The figure shows three views and two pictorial views of one solid part (mm, origin at its lowest corner). Answer the questions. A direction names the side the tool comes from. Coordinates: 2 decimals unless noted, no trailing zeros. Order: outer loops, then holes, each group sorted by start corner. A loop starts at its lowest first (then second) coordinate and runs counter-clockwise, first axis right, second up. Notation, with made-up numbers: (-35.75, 58.5) -> (10.25, 58.5) arc R29 cw to (10.25, 89.5) -> close; hole circle Ø8 at (-15.75, 75.5). An arc over 180 degrees is marked (long way). Return JSON: item names as keys, results as strings.
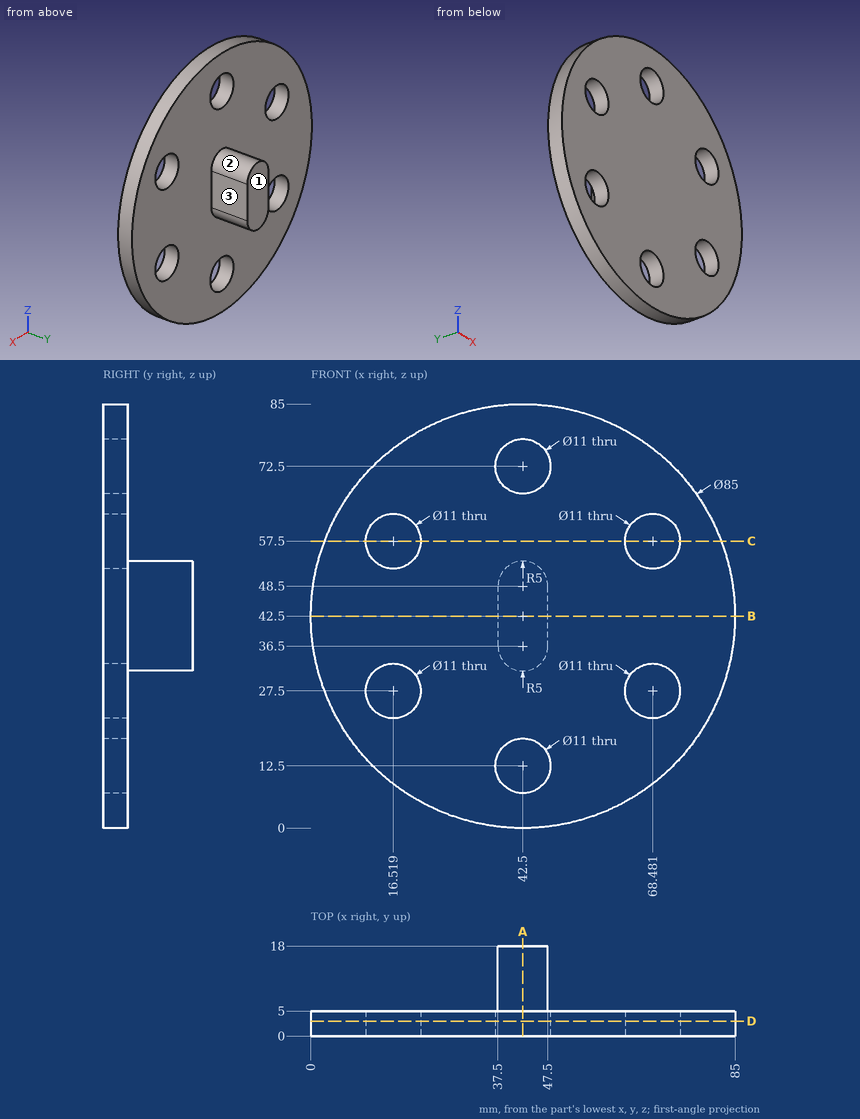
Item 1: The part is cut by section A-A on x = 42.5. Determine the outline of the cut face in (y, z), plus the area to 3 significant figures.
Answer list:
{"outline": "(0, 0) -> (5, 0) -> (5, 7) -> (0, 7) -> close; (0, 18) -> (5, 18) -> (5, 31.5) -> (18, 31.5) -> (18, 53.5) -> (5, 53.5) -> (5, 67) -> (0, 67) -> close; (0, 78) -> (5, 78) -> (5, 85) -> (0, 85) -> close", "area": "601 mm2"}
Item 2: The part is cut by section B-B on z = 42.5. Determine the outline of the cut face in (x, y), plus the area to 3 significant figures.
Answer list:
{"outline": "(0, 0) -> (85, 0) -> (85, 5) -> (47.5, 5) -> (47.5, 18) -> (37.5, 18) -> (37.5, 5) -> (0, 5) -> close", "area": "555 mm2"}
Item 3: The part is cut by section D-D on y = 3. Determine the outline of the cut face in (x, z), plus the area to 3 significant figures.
Answer list:
{"outline": "circle Ø85 at (42.5, 42.5); hole circle Ø11 at (16.52, 27.5); hole circle Ø11 at (16.52, 57.5); hole circle Ø11 at (42.5, 12.5); hole circle Ø11 at (42.5, 72.5); hole circle Ø11 at (68.48, 27.5); hole circle Ø11 at (68.48, 57.5)", "area": "5,100 mm2"}
Item 4: The part is cut by section C-C on z = 57.5. Determine the outline of the cut face in (x, y) (1 decimal).
Answer list:
{"outline": "(2.7, 0) -> (11, 0) -> (11, 5) -> (2.7, 5) -> close; (22, 0) -> (63, 0) -> (63, 5) -> (22, 5) -> close; (74, 0) -> (82.3, 0) -> (82.3, 5) -> (74, 5) -> close"}
Item 5: Flat-ended cylindrical pins translate along their axes: pin 1 (8 mm diameter, centred on y = 3, z = 69, fed in from -X) (1 decimal); pin 2 (6 mm diameter, centred on y = 12.5, z = 42.5, fed in from +X); pin 3 (5 mm diameter, centred on y = 13, z = 58, fed in from +X); pin 4 (6 mm diameter, centred on x = 45, z = 68, fed in from +Y). Find the tip coordinate at first contact, or state that the pin passes through.
Answer list:
{"pin 1": "x = 6.4", "pin 2": "x = 47.5", "pin 3": "through", "pin 4": "y = 5"}
Item 6: Find the intervals of material crossed by probe 1 along X at (y, z) = (3.25, 57.5) (1 decimal); probe 2 along Y at (x, z) = (62, 51); probe 3 along X at (y, z) = (4.5, 77), in increasing order.
Answer list:
{"probe 1": "2.7 to 11, 22 to 63, 74 to 82.3", "probe 2": "0 to 5", "probe 3": "17.68 to 39.34, 45.66 to 67.32"}
Item 7: Which of the six approach directions +Z, -Z, +X, -X, +Y, -Y give full straight-line access (tool end or side, diameter ignored) to the marked faces 1, 2 and 3?
Answer list:
{"face 1": "+Z, -Z, +X, -X, +Y", "face 2": "+Z, +Y", "face 3": "+Z, -Z, +X, +Y"}
